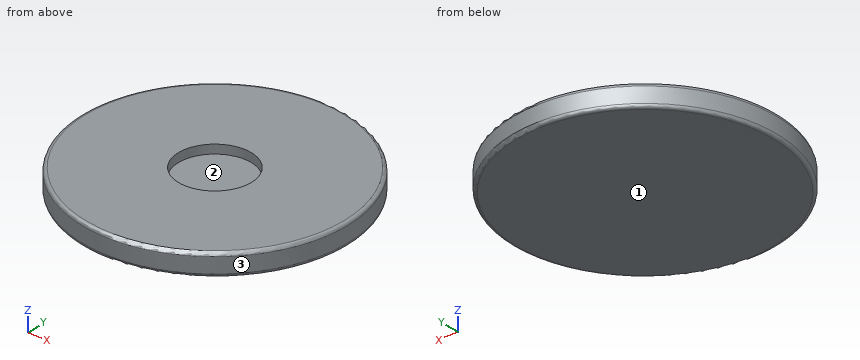
from build123d import *

# Parameters (mm, degrees)
F0_R     = 6
F1_DEPTH = 1
F2_R     = 0.15
F3_R     = 1.65
F4_DEPTH = 0.4


# Not quite as in the source:
# - a feature names something its author has since deleted; it is built from what else it names


with BuildPart() as f1:
    # F0 (on Top) → F1 (new body)
    with BuildSketch(Plane.XY):
        Circle(F0_R)
    extrude(amount=F1_DEPTH)

    # F2
    f2_edges = [f1.edges().sort_by_distance(p)[0] for p in [
        (-6, 0, 1),
        (-6, 0, 0),
    ]]
    fillet(f2_edges, radius=F2_R)

    # F3 (on face) → F4 (cut)
    with BuildSketch(Plane.XY.offset(1)):
        Circle(F3_R)
    extrude(amount=-F4_DEPTH, mode=Mode.SUBTRACT)


solid = f1.part
Here's how the part is built. I have some questions about the finished solid (model axes, mm). Face numbers are marked on the shaded views. Give positions to 0.01 mm unless a question says otherwise; leave off trailing zeros. Write each loop counter-clockwise with the first axis right and the second up, starting at its lowest first coordinate (ties: lowest second). Pieces come first, ordered by that corner, then holes. Notation, with made-up numbers: (37.5, 35.25) -> (43.5, 35.25) arc R23 ccw to (43.5, 57.25) -> close; hole circle Ø10 at (29.25, 12.5). An arc over 180 degrees is marked (long way). Use one line per item in the form item = value. Start each with the question number.
1. If I drill on L1, parallel to Y at x = 0, z = 0.8; L2, parallel to X at y = -0.25, z = 0.8; L3, parallel to Y at x = -1, z = 0.5, over which ranges is the centre line in solid material (lowest first)?
2. Imagine slicing it at C-C on z = 0.4. List the corners of the cut face in (x, y) for me.
3. Thinking about a two-plate mould opening in X: for the marked faces 1, 2 and 3, which applies, +X half, -X half, draft (parallel to the pull), parting line (faces both ways), or undercut?
4. Imagine slicing it at A-A on x = 0. List the corners of the cut face in (y, z) for me.
Entries:
q1.L1 = -6 to -1.65, 1.65 to 6
q1.L2 = -5.99 to -1.63, 1.63 to 5.99
q1.L3 = -5.92 to 5.92
q2.outline = circle Ø12 at (0, 0)
q3.face_1 = draft
q3.face_2 = undercut
q3.face_3 = parting line
q4.outline = (-6, 0.15) arc R0.15 ccw to (-5.85, 0) -> (5.85, 0) arc R0.15 ccw to (6, 0.15) -> (6, 0.85) arc R0.15 ccw to (5.85, 1) -> (1.65, 1) -> (1.65, 0.6) -> (-1.65, 0.6) -> (-1.65, 1) -> (-5.85, 1) arc R0.15 ccw to (-6, 0.85) -> close
